CAD build for the part. Positions are in the model's coordinates, mm. A direction names the side the tool comes from. Round coordinates to 2 decimals unless told otherwise and drop trailing zeros. Loops run counter-clockwise (first coordinate to the right, second up) from the corner with the lowest first, then second, coordinate; pieces in that order, holes last. Notation, with made-up numbers: M 61.5,-11 L 78.5,-11 A9 ccw 78.5,-7 Z; hole C 21,29.25 d11. An arc over 180 degrees is marked long. Use one line per item in the form item = value.
Autodesk Fusion 360 part; units mm, degrees
sketch "Sketch1" plane through (0, 0, 0) normal (0, 1, 0) x (1, 0, 0)
  line L0 (75, -25) -> (-75, -25)
  line L1 (-75, -25) -> (-75, 25)
  line L2 (-75, 25) -> (75, 25)
  line L3 (75, 25) -> (75, -25)
  line L4 (75, -25) -> (-75, 25) construction
  line L5 (-75, -25) -> (75, 25) construction
  dimension "d1" = 150
  dimension "d2" = 50
extrude "Extrude1" add sketch "Sketch1" along normal blind 65
sketch "Sketch2" plane through (0, 0, 25) normal (0, 0, 1) x (1, 0, 0)
  line L0 (-75, 0) -> (75, 0)
  line L1 (75, 0) -> (75, 65)
  line L2 (75, 65) -> (-75, 65)
  line L3 (-75, 65) -> (-75, 0)
  line L4 (-75, 0) -> (75, 0)
  line L5 (75, 0) -> (75, 15)
  line L6 (75, 15) -> (-75, 15)
  line L7 (-75, 15) -> (-75, 0)
  line L8 (-75, 65) -> (-50, 65)
  line L9 (-50, 65) -> (-50, 15)
  line L10 (-50, 15) -> (-75, 15)
  line L11 (-75, 15) -> (-75, 65)
  line L12 (75, 65) -> (50, 65)
  line L13 (50, 65) -> (50, 15)
  line L14 (50, 15) -> (75, 15)
  line L15 (75, 15) -> (75, 65)
  line L16 (-50, 65) -> (-30, 65)
  line L17 (-30, 65) -> (-30, 15)
  line L18 (-30, 15) -> (-50, 15)
  line L19 (-50, 15) -> (-50, 65)
  line L20 (-30, 65) -> (-10, 65)
  line L21 (-10, 65) -> (-10, 15)
  line L22 (-10, 15) -> (-30, 15)
  line L23 (-30, 15) -> (-30, 65)
  line L24 (-10, 65) -> (10, 65)
  line L25 (10, 65) -> (10, 15)
  line L26 (10, 15) -> (-10, 15)
  line L27 (-10, 15) -> (-10, 65)
  line L28 (10, 65) -> (30, 65)
  line L29 (30, 65) -> (30, 15)
  line L30 (30, 15) -> (10, 15)
  line L31 (10, 15) -> (10, 65)
  line L32 (30, 65) -> (50, 65)
  line L33 (50, 65) -> (50, 15)
  line L34 (50, 15) -> (30, 15)
  line L35 (30, 15) -> (30, 65)
  dimension "d5" = 150
  dimension "d6" = 15
  dimension "d7" = 20
  dimension "d8" = 20
  dimension "d9" = 20
  dimension "d10" = 20
  dimension "d11" = 20
  dimension "d12" = 25
extrude "Extrude2" cut sketch "Sketch2" against normal blind 50 contours L2 L6 L9 L16 L17 L18 L19 L23 | L2 L6 L13 L29 L32 L33 L34 L35 | L2 L6 L21 L24 L25 L26 L27 L31
sketch "Sketch3" plane through (-75, 0, 0) normal (-1, 0, 0) x (0, 0, 1)
  line L0 (-25, 0) -> (25, 0)
  line L1 (25, 0) -> (25, 65)
  line L2 (25, 65) -> (-25, 65)
  line L3 (-25, 65) -> (-25, 0)
  circle A0 centre (0, 40) radius 25
  dimension "d15" = 40
extrude "Extrude3" cut sketch "Sketch3" against normal blind 150 contours L2 L3 A0 | L1 L2 A0
sketch "Sketch4" plane through (0, 15, 0) normal (0, 1, 0) x (-1, 0, 0)
  line L0 (50, 25) -> (30, 25)
  line L1 (30, 25) -> (30, -25)
  line L2 (30, -25) -> (50, -25)
  line L3 (50, -25) -> (50, 25)
  circle A0 centre (40, 0) radius 5
  circle A1 centre (0, 0) radius 5
  circle A2 centre (-40, 0) radius 5
hole "Hole1" at (-40, 15, 0) at (0, 15, 0) at (40, 15, 0) direction (0, -1, 0) diameter 10 depth 30 tip angle 118 counterbore diameter 16 counterbore depth 10
sketch "Sketch5" plane through (-75, 0, 0) normal (-1, 0, 0) x (0, 0, 1)
  arc A0 (25, 40) -> (-25, 40) centre (0, 40) ccw
  line L0 (-25, 40) -> (-25, 0)
  line L1 (-25, 0) -> (25, 0)
  line L2 (25, 0) -> (25, 40)
  circle A1 centre (0, 40) radius 25
  dimension "d23" = 50
hole "Hole2" at (-75, 40, 0) direction (1, 0, 0) diameter 25 depth 150 tip angle 180
1. Cut at A-A on y = 21.5. Write the cut outline in (x, z), and give its area (3 significant figures).
Completed:
outline = M -75,-25 L -50,-25 L -50,25 L -75,25 Z; M -30,-25 L -10,-25 L -10,25 L -30,25 Z; M 10,-25 L 30,-25 L 30,25 L 10,25 Z; M 50,-25 L 75,-25 L 75,25 L 50,25 Z
area = 4,500 mm2
2. Cut at C-C on x = -14.5. Write the cut outline in (y, z), and give its area (3 significant figures).
Completed:
outline = M 0,-25 L 40,-25 A25 ccw 40,25 L 0,25 Z; hole C 40,0 d25
area = 2,490 mm2
3. Probe line 1 along X through (y, z) = (10, 0); line 2 along X through (y, z) = (3, 0); line 3 along Z through (x, y) = (0, 10). List the from-to ranges inside material, lowest first. Write a range as from..to.
Completed:
line_1 = -75..-48, -32..-8, 8..32, 48..75
line_2 = -75..-45, -35..-5, 5..35, 45..75
line_3 = -25..-8, 8..25
4. Cut at B-B on x = -40. Write the cut outline in (y, z).
Completed:
outline = M 0,-25 L 15,-25 L 15,-8 L 5,-8 L 5,-5 L 0,-5 Z; M 0,5 L 5,5 L 5,8 L 15,8 L 15,25 L 0,25 Z
5. Tool access for faces 4 (the face through (-44.957, 2.465, -0.651)), 5 (the face through (32.068, 9.93, -1.041)), 6 (the face through (-10, 24, 0)): list every direction of +Z, -Z, +X, -X, +Y, -Y with a clear straight run to the whole face (end or side of a thin tool).
Completed:
face_4 = +Y, -Y
face_5 = +Y
face_6 = +Z, -Z, +Y
6. Cut at D-D on y = 47.5. State how many separate pieces and enclosed holes the cut face has, and give its area (3 significant figures).
Completed:
separate_pieces = 8
enclosed_holes = 0
area = 2,490 mm2
7. Drop flat-ended pins along their axis: P1, Ø1.5, axis at x = -36.5, z = 10, coming from the +Y side; P2, Ø13, axis at x = 40, z = 0, coming from the -Y side; P3, Ø13, axis at x = 40, z = 0, coming from the +Y side; P4, Ø5, axis at x = 31, y = 49.5, coming from the -Z side. Give the stop position or say it passes through.
Completed:
P1 = 15
P2 = 0
P3 = 5
P4 = -23.94
8. Pull direction Z, two halves, no side cores. Call faces 1 (the face through (4.88, 2.46, -1.08)), 2 (the face through (1, 11, 25)), 3 (the face through (-75, 25, 0)): +Z half, -Z half, draft (parallel to the pull), parting line (faces both ways), or undercut.
Completed:
face_1 = undercut
face_2 = +Z half
face_3 = draft
